The model under review builds one solid part; all positions refer to its coordinate system, in mm. A direction names the side the tool comes from. Round coordinates to 2 decimals unless told otherwise and drop trailing zeros. Loops run counter-clockwise (first coordinate to the right, second up) from the corner with the lowest first, then second, coordinate; pieces in that order, holes last. Notation, with made-up numbers: M -13.75,28 L 0.25,28 A24 cw 0.25,53 Z; hole C 5,19.5 d3. An arc over 180 degrees is marked long. Use a Markdown table: item, result. Add a question column.
```python
from build123d import *

# Parameters (mm, degrees)
SKETCH_1_R               = 8.5
SKETCH_1_R_2             = 6.7
EXTRUDE_1_DEPTH          = 8.5
SKETCH_2_W               = 1.3
SKETCH_2_H               = 1.1
SKETCH_4_W               = 3.6
SKETCH_4_H               = 17
CUT_EXTRUDE_1_DEPTH      = 8.5
PATTERN_START            = 3
PATTERN_CIRCULAR_1_DEPTH = 5.5000001


# Read off the part's stored shape, not the designer's step: Круговой массив1
with BuildPart() as part:
    # Эскиз1 → Вытянуть1 (new body)
    with BuildSketch(Plane(origin=(0, 0, 0), x_dir=(0, 0, -1), z_dir=(1, 0, 0))):
        Circle(SKETCH_1_R)
        Circle(SKETCH_1_R_2, mode=Mode.SUBTRACT)
    extrude(amount=EXTRUDE_1_DEPTH)

    # Эскиз2 → Вырез-Повернуть1 (revolve, cut)
    with BuildSketch(Plane.XY, mode=Mode.PRIVATE) as cut_revolve_1_sk:
        with Locations((3.65, 7.95)):
            Rectangle(SKETCH_2_W, SKETCH_2_H)
    revolve(cut_revolve_1_sk.sketch.rotate(Axis((8.5, 0, 0), (-1, 0, 0)), 90), axis=Axis((8.5, 0, 0), (-1, 0, 0)), mode=Mode.SUBTRACT)

    # Эскиз3 → Вырез-Повернуть2 (revolve, cut)
    with BuildSketch(Plane.XY, mode=Mode.PRIVATE) as cut_revolve_2_sk:
        Polygon((8.5, 6.7), (6.7, 8.5), (8.5, 8.5), align=None)
    revolve(cut_revolve_2_sk.sketch.rotate(Axis((8.5, 0, 0), (-1, 0, 0)), 90), axis=Axis((8.5, 0, 0), (-1, 0, 0)), mode=Mode.SUBTRACT)

    # Эскиз4 → Вырез-Вытянуть1 (cut)
    with BuildSketch(Plane(origin=(3, 0, 0), x_dir=(0, 0, -1), z_dir=(1, 0, 0))):
        Rectangle(SKETCH_4_W, SKETCH_4_H)
    extrude(amount=CUT_EXTRUDE_1_DEPTH, mode=Mode.SUBTRACT)

    # Круговой массив1 outline → Круговой массив1 (cut)
    with BuildSketch(Plane.YZ.offset(PATTERN_START)):
        with BuildLine():
            ThreePointArc((4.785686287, -4.689051798), (3.35, -5.802370205), (1.667994833, -6.489051798))
            Line((1.667994833, -6.489051798), (2.594767158, -8.094268552))
            ThreePointArc((2.594767158, -8.094268552), (4.25, -7.361215932), (5.712458612, -6.294268552))
            Line((5.712458612, -6.294268552), (4.785686287, -4.689051798))
        make_face()
        with BuildLine():
            ThreePointArc((-1.667994833, -6.489051798), (-3.35, -5.802370205), (-4.785686287, -4.689051798))
            Line((-4.785686287, -4.689051798), (-5.712458612, -6.294268552))
            ThreePointArc((-5.712458612, -6.294268552), (-4.25, -7.361215932), (-2.594767158, -8.094268552))
            Line((-2.594767158, -8.094268552), (-1.667994833, -6.489051798))
        make_face()
        with BuildLine():
            ThreePointArc((1.667994833, 6.489051798), (3.35, 5.802370205), (4.785686287, 4.689051798))
            Line((4.785686287, 4.689051798), (5.712458612, 6.294268552))
            ThreePointArc((5.712458612, 6.294268552), (4.25, 7.361215932), (2.594767158, 8.094268552))
            Line((2.594767158, 8.094268552), (1.667994833, 6.489051798))
        make_face()
        with BuildLine():
            ThreePointArc((-4.785686287, 4.689051798), (-3.35, 5.802370205), (-1.667994833, 6.489051798))
            Line((-1.667994833, 6.489051798), (-2.594767158, 8.094268552))
            ThreePointArc((-2.594767158, 8.094268552), (-4.25, 7.361215932), (-5.712458612, 6.294268552))
            Line((-5.712458612, 6.294268552), (-4.785686287, 4.689051798))
        make_face()
    extrude(amount=PATTERN_CIRCULAR_1_DEPTH, mode=Mode.SUBTRACT)


solid = part.part
```
(1) Insertion check: pin 1 Ø1 at (x, y) = (5, 3) entering from -Z; pin 2 Ø1.5 at (x, z) = (5, -0.5) entering from +Y; pin 3 Ø2 at (x, y) = (6, 7) entering from -Z; pin 4 Ø0.9 at (x, y) = (5.5, 7.5) entering from +Z. Each pin has a flat end and moves straight along its axis. Give the tip position at first contact, or say it passes through.
(2) Draft analysis for pull direction Z (two halves, no side actions). For faces 1 (the face through (5.71, 2.03, 7.12)), 2 (the face through (5.5, 0, -8.5)), 3 (the face through (5.5, 0, 8.5)), state which applies: released by +Z, released by -Z, zero draft, split by the parting line, or undercut.
(3) Consider section A-A, the plane z = 0. Give the boundary of the cut face in (x, y), then the cut area to 3 significant figures.
(4) To check wall thickness, follow probe 1 along Z at (x, y) = (5.75, 0); probe 2 along X at (y, z) = (-6.75, 1.75); probe 3 along Z at (x, y) = (3.5, 6.75). State the ranges of each line that lie inside material, in increasing order.
(5) For faces 4 (the face through (4.3, -7, 4)), 5 (the face through (4.3, 7, 4)), 6 (the face through (3.659, -6.394, -3.725)), 7 (the face through (5.71, 5.15, -5.32)), list the 3-axis set-ups (+Z, -Z, +X, -X, +Y, -Y) from which the entire face can be reached by the end or side of a thin tool; tool diameter is ignored.
(6) Consider section C-C, the plane x = 2. Give the boundary of the cut face in (y, z), then the cut area to 3 significant figures.
(7) Consider section D-D, the plane y = 4. Give the boundary of the cut face in (x, z).
(8) Consider section B-B, the plane y = 0. Give the boundary of the cut face in (x, z), then the cut area to 3 significant figures.
Found:
| question | item | result |
|---|---|---|
| 1 | pin 1 | stops at z = -8.12 |
| 1 | pin 2 | passes through |
| 1 | pin 3 | stops at z = -6.02 |
| 1 | pin 4 | stops at z = 4.75 |
| 2 | face 1 | undercut |
| 2 | face 2 | released by -Z |
| 2 | face 3 | released by +Z |
| 3 | outline | M 0,-8.5 L 3,-8.5 L 3,-6.7 L 0,-6.7 Z; M 0,6.7 L 3,6.7 L 3,8.5 L 0,8.5 Z |
| 3 | area | 10.8 mm^2 |
| 4 | probe 1 | z = -8.5 to -6.7, 6.7 to 8.5 |
| 4 | probe 2 | x = 0 to 3 |
| 4 | probe 3 | z = -3.03 to -1.8, 1.8 to 3.03 |
| 5 | face 4 | +Z, -Y |
| 5 | face 5 | +Z, +Y |
| 5 | face 6 | -Z, -Y |
| 5 | face 7 | -Z, +X |
| 6 | outline | C 0,0 d17; hole C 0,0 d13.4 |
| 6 | area | 86.0 mm^2 |
| 7 | outline | M 0,-7.5 L 3,-7.5 L 3,-5.37 L 0,-5.37 Z; M 0,5.37 L 3,5.37 L 3,7.5 L 0,7.5 Z |
| 8 | outline | M 0,-8.5 L 3,-8.5 L 3,-7.4 L 4.3,-7.4 L 4.3,-8.5 L 6.7,-8.5 L 8.5,-6.7 L 0,-6.7 Z; M 0,6.7 L 8.5,6.7 L 6.7,8.5 L 4.3,8.5 L 4.3,7.4 L 3,7.4 L 3,8.5 L 0,8.5 Z |
| 8 | area | 24.5 mm^2 |
